Input: part model. Units: mm. Frame: model coordinates. A direction names the side the tool comes from. Round coordinates to 2 decimals unless told otherwise and drop trailing zeros. Loops run counter-clockwise (first coordinate to the right, second up) from the corner with the lowest first, then second, coordinate; pieces in that order, holes last. Notation, with made-up numbers: M 1.25,0.5 L 37.25,0.5 A29 cw 37.25,26.5 Z; hole C 85,57 d3. An arc over 180 degrees is marked long. Use one line per item in the form item = value. Start each with the question number.
Q1. Mould query, pull axis Z, two halves, no side actions, for faces 1 (the flat face through (31, 10.16, 14)), 2 (the flat face through (10.16, 30, 14)), 3 (the flat face through (2, 13, 184.15)), 4 (the flat face through (25.4, 13, 108)). Classes: pulls with the +Z half, pulls with the -Z half, needs draft (parallel to the pull), parting line crosses it, or undercut.
Q2. Section query A-A, the plane x = 42. Output: boundary loops of the cut face in (y, z).
Q3. Access query for faces 5 (the flat face through (13, 13, 181.61)), 6 (the flat face through (31, 31, 23.368)), 7 (the flat face through (31, 31, 31.75)), 8 (the flat face through (13, 25.4, 108)). Directions: +Z, -Z, +X, -X, +Y, -Y. A direction counts if a zero-diameter tool reaches every point of the face in a straight line with its end or side. Return the directions, or none.
Q4. Section query C-C, the plane z = 16.5. Output: boundary loops of the cut face in (x, y), and give its area (3 significant figures).
Q5. Ray query, line 1 along Z through (x, y) = (18.5, 11); line 2 along Z through (x, y) = (36, 40.5); line 3 along Y through (x, z) = (22.5, 8). Return the intervals inside material, ascending.
Q6. First-contact query: P1, Ø10, axis at y = 40, z = 10, coming from the +X side; P2, Ø10, axis at x = 41, y = 37.5, coming from the -Z side; P3, Ø20.5, axis at y = 17, z = 85, coming from the +X side. Flat tips, straight axial feed; report the tip coordinate or a pass-through.
Q7. Section query D-D, the plane z = 75. Output: boundary loops of the cut face in (x, y), and give its area (3 significant figures).
Autodesk Fusion 360 part; units mm, degrees
sketch "Sketch1" plane through (0, 0, 0) normal (0, 0, 1) x (1, 0, 0)
  line L0 (0, 0) -> (50.8, 0)
  line L1 (50.8, 0) -> (50.8, 50.8)
  line L2 (50.8, 50.8) -> (0, 50.8)
  line L3 (0, 50.8) -> (0, 0)
  dimension "d1" = 50.8
  dimension "d2" = 50.8
extrude "Extrude1" add sketch "Sketch1" along normal blind 31.75
sketch "Sketch2" plane through (50.8, 0, 0) normal (1, 0, 0) x (0, 1, 0)
  line L0 (0, 0) -> (50.8, 0)
  line L1 (50.8, 0) -> (50.8, 31.75)
  line L2 (50.8, 31.75) -> (0, 31.75)
  line L3 (0, 31.75) -> (0, 0)
  line L4 (50.8, 23.368) -> (10.16, 23.368)
  line L5 (10.16, 23.368) -> (10.16, 3.81)
  line L6 (10.16, 3.81) -> (50.8, 3.81)
  line L7 (50.8, 3.81) -> (50.8, 23.368)
  dimension "d5" = 40.64
  dimension "d6" = 19.558
  dimension "d14" = 3.81
extrude "Extrude2" cut sketch "Sketch2" against normal blind 40.64 contours L1 L4 L5 L6 L7
sketch "Sketch3" plane through (0, 0, 31.75) normal (0, 0, 1) x (-1, 0, 0)
  line L0 (0, -50.8) -> (0, 0)
  line L1 (0, 0) -> (-50.8, 0)
  line L2 (-50.8, 0) -> (-50.8, -50.8)
  line L3 (-50.8, -50.8) -> (0, -50.8)
  line L4 (0, 0) -> (-25.4, 0)
  line L5 (-25.4, 0) -> (-25.4, -25.4)
  line L6 (-25.4, -25.4) -> (0, -25.4)
  line L7 (0, -25.4) -> (0, 0)
  dimension "d10" = 25.4
  dimension "d11" = 25.4
extrude "Extrude3" add sketch "Sketch3" along normal blind 152.4 contours L0 L1 L4 L5 L6 L7
fillet "Fillet1" radius 2.54 2 edges at (25.4, 12.7, 31.75) (12.7, 25.4, 31.75)
sketch "Sketch4" plane through (0, 0, 0) normal (0, 0, -1) x (1, 0, 0)
  line L0 (0, 0) -> (0, -50.8)
  line L1 (0, -50.8) -> (50.8, -50.8)
  line L2 (50.8, -50.8) -> (50.8, 0)
  line L3 (50.8, 0) -> (0, 0)
  line L4 (2.54, -2.54) -> (22.86, -2.54)
  line L5 (22.86, -2.54) -> (22.86, -22.86)
  line L6 (22.86, -22.86) -> (2.54, -22.86)
  line L7 (2.54, -22.86) -> (2.54, -2.54)
  dimension "d17" = 2.54
  dimension "d18" = 2.54
  dimension "d19" = 20.32
  dimension "d20" = 20.32
sketch "Sketch5" plane through (0, 0, 0) normal (0, 0, -1) x (1, 0, 0)
  line L0 (5.334, -5.334) -> (20.066, -5.334)
  line L1 (20.066, -5.334) -> (20.066, -20.066)
  line L2 (20.066, -20.066) -> (5.334, -20.066)
  line L3 (5.334, -20.066) -> (5.334, -5.334)
  line L4 (0, -50.8) -> (0, 0)
  line L5 (0, 0) -> (50.8, 0)
  dimension "d37" = 14.732
  dimension "d38" = 14.732
  dimension "d39" = 5.334
  dimension "d40" = 5.334
sketch "Sketch6" plane through (0, 0, 184.15) normal (0, 0, 1) x (-1, 0, 0)
  line L0 (0, -25.4) -> (0, 0)
  line L1 (0, 0) -> (-25.4, 0)
  line L2 (-25.4, 0) -> (-25.4, -25.4)
  line L3 (-25.4, -25.4) -> (0, -25.4)
  line L4 (-2.54, -22.86) -> (-22.86, -22.86)
  line L5 (-22.86, -22.86) -> (-22.86, -2.54)
  line L6 (-22.86, -2.54) -> (-2.54, -2.54)
  line L7 (-2.54, -2.54) -> (-2.54, -22.86)
  line L8 (-5.08, -20.32) -> (-20.32, -20.32)
  line L9 (-20.32, -20.32) -> (-20.32, -5.08)
  line L10 (-20.32, -5.08) -> (-5.08, -5.08)
  line L11 (-5.08, -5.08) -> (-5.08, -20.32)
  dimension "d27" = 2.54
  dimension "d28" = 2.54
  dimension "d29" = 2.54
  dimension "d30" = 20.32
  dimension "d31" = 2.54
  dimension "d32" = 15.24
  dimension "d33" = 15.24
  dimension "d34" = 2.54
extrude "Extrude5" cut sketch "Sketch6" against normal blind 2.54 contours L8 L9 L10 L11
loft "Loft2" cut profiles "Sketch6" section 1 contours L4 L5 L6 L7 section 2 face at (15.24, 15.24, 181.61)
extrude "Extrude7" add sketch "Sketch5" along normal blind 2.54
loft "Loft3" add profiles "Sketch4" section 1 contours L4 L5 L6 L7 section 2 face at (15.1553, 10.2447, -2.54)
Results found:
q1.face_1 = undercut
q1.face_2 = undercut
q1.face_3 = pulls with the +Z half
q1.face_4 = needs draft
q2.outline = M 0,0 L 50.8,0 L 50.8,3.81 L 10.16,3.81 L 10.16,23.37 L 50.8,23.37 L 50.8,31.75 L 0,31.75 Z
q3.face_5 = +Z
q3.face_6 = +X, +Y
q3.face_7 = +Z, +X, +Y
q3.face_8 = +Z, +X, -X, +Y
q4.outline = M 0,0 L 50.8,0 L 50.8,10.16 L 10.16,10.16 L 10.16,50.8 L 0,50.8 Z
q4.area = 929 mm²
q5.line_1 = -2.54 to 3.81, 23.37 to 181.61
q5.line_2 = 0 to 3.81, 23.37 to 31.75
q5.line_3 = 0 to 10.16
q6.P1 = 10.16
q6.P2 = 0
q6.P3 = 25.4
q7.outline = M 0,0 L 25.4,0 L 25.4,25.4 L 0,25.4 Z
q7.area = 645 mm²
